from build123d import *

# Parameters (mm, degrees)
F0_W            = 12.2174
F0_H            = 38.1762
F1_DEPTH        = 117.475
F2_W            = 2.286
F2_H            = 1.778
F3_DEPTH        = 117.476
F5_DEPTH        = 117.476
F7_D            = 2.7051
F10_D           = 2.7051
F10_DEPTH       = 5.55625
F10_TIP         = 0.8126940303
F10_ON_F9_D     = 2.7051
F10_ON_F9_DEPTH = 5.55625
F10_ON_F9_TIP   = 0.8126940303


with BuildPart() as f1:
    # F0 (on Front) → F1 (new body)
    with BuildSketch(Plane.XZ):
        with Locations((6.1087, 19.0881)):
            Rectangle(F0_W, F0_H)
    extrude(amount=F1_DEPTH)

    # F2 (on face) → F3 (cut, through all)
    with BuildSketch(Plane.XZ.offset(117.475)):
        with Locations((1.143, 29.5021)):
            Rectangle(F2_W, F2_H)
        with Locations((1.143, 25.6921)):
            Rectangle(F2_W, F2_H)
        with Locations((1.143, 8.6741)):
            Rectangle(F2_W, F2_H)
        with Locations((1.143, 12.4841)):
            Rectangle(F2_W, F2_H)
    extrude(amount=-F3_DEPTH, mode=Mode.SUBTRACT)

    # F4 (on face) → F5 (cut, through all)
    with BuildSketch(Plane.XZ.offset(117.475)):
        Polygon((10.5664, 20.3581), (12.2174, 20.3581), (12.2174, 38.1762), (7.1374, 38.1762), (7.1374, 36.6522), (10.5664, 36.6522), (10.5664, 24.8031), (5.8674, 24.8031), (5.8674, 22.2631), (10.5664, 22.2631), align=None)
        Polygon((10.5664, 13.3731), (10.5664, 1.524), (7.1374, 1.524), (7.1374, 0), (12.2174, 0), (12.2174, 17.8181), (10.5664, 17.8181), (10.5664, 15.9131), (5.8674, 15.9131), (5.8674, 13.3731), align=None)
    extrude(amount=-F5_DEPTH, mode=Mode.SUBTRACT)

    # F7 (through all)
    with Locations(Plane.XZ.offset(117.475)):
        with Locations((3.2004, 34.9631), (3.2004, 3.2131)):
            Hole(F7_D / 2)

    # F10
    with Locations(Plane.YZ.offset(10.5664)):
        with Locations((-101.6, 28.3083), (-15.875, 28.3083)):
            Hole(F10_D / 2, depth=F10_DEPTH)
            with Locations((0, 0, -(F10_DEPTH + F10_TIP / 2))):  # 118° drill point
                Cone(0, F10_D / 2, F10_TIP, mode=Mode.SUBTRACT)

    # F10 on F9
    with Locations(Plane.YZ.offset(10.5664)):
        with Locations((-15.875, 9.8679), (-101.6, 9.8679)):
            Hole(F10_ON_F9_D / 2, depth=F10_ON_F9_DEPTH)
            with Locations((0, 0, -(F10_ON_F9_DEPTH + F10_ON_F9_TIP / 2))):  # 118° drill point
                Cone(0, F10_ON_F9_D / 2, F10_ON_F9_TIP, mode=Mode.SUBTRACT)


solid = f1.part
Part model, mm, in its own coordinate system. A direction names the side the tool comes from. Coordinates: 2 decimals unless noted, no trailing zeros. Order: outer loops, then holes, each group sorted by start corner. A loop starts at its lowest first (then second) coordinate and runs counter-clockwise, first axis right, second up. Notation, with made-up numbers: M 61,81 L 108,81 A24 ccw 108,100 Z; hole C -17,53.5 d10. An arc over 180 degrees is marked long. One line per question, with ' | ' between items.
Q1. Two-plate mould, pull along Z, no slides. Class faces 6 (the face through (10.566, -60, 31)), 7 (the face through (3.49, -57.92, 1.89)), 8 (the face through (4, -58, 0)): +Z half, -Z half, draft (parallel to the pull), parting line (faces both ways), or undercut.
A:
face 6: draft | face 7: undercut | face 8: -Z half
Q2. 3-axis set-ups, long thin cutter, end or side, ignore diameter. For faces 1 (the face through (7.749, -14.524, 9.927)), 2 (the face through (9, -60, 1.524)), 3 (the face through (8, -60, 24.803)), 4 (the face through (9, -60, 36.652)), 5 (the face through (1, -60, 28.613)): which of +Z, -Z, +X, -X, +Y, -Y reach the whole face in a straight line?
A:
face 1: +X | face 2: -Z, +X, +Y, -Y | face 3: +X, +Y, -Y | face 4: +Z, +X, +Y, -Y | face 5: -X, +Y, -Y
Q3. Slice it at A-A (x = 8.25). Give the cut face in (y, z) (3 decimals).
A:
outline: M -117.475,1.524 L 0,1.524 L 0,13.373 L -117.475,13.373 Z; M -117.475,15.913 L 0,15.913 L 0,22.263 L -117.475,22.263 Z; M -117.475,24.803 L 0,24.803 L 0,36.652 L -117.475,36.652 Z; hole C -101.6,9.868 d2.705; hole C -101.6,28.308 d2.705; hole C -15.875,9.868 d2.705; hole C -15.875,28.308 d2.705
Q4. Drill centre lines: line 1 (Z direction, x = 7, y = -9); line 2 (Z direction, x = 1.5, y = -24); line 3 (Z direction, x = 8.5, y = -59.5). Where is each one in solid material? Low to high.
A:
line 1: z = 0 to 13.37, 15.91 to 22.26, 24.8 to 38.18 | line 2: z = 0 to 7.79, 9.56 to 11.6, 13.37 to 24.8, 26.58 to 28.61, 30.39 to 38.18 | line 3: z = 1.52 to 13.37, 15.91 to 22.26, 24.8 to 36.65
Q5. Slice it at B-B (y = -99). Count the separate pieces of the cut face and the enclosed holes in it, and give its area (3 significant figures).
A:
separate pieces: 1 | enclosed holes: 2 | area: 346 mm^2
Q6. Pin check, flat tips, straight feed: P1, Ø4, axis at x = 6, z = 18.5, coming from the +Y side; P2, Ø0.8, axis at y = -65.5, z = 38, coming from the +X side; P3, Ø1.6, axis at x = 3.2, z = 34.96, coming from the -Y side; P4, Ø0.8, axis at y = -77.5, z = 14, coming from the +X side. Stop position of each tip, or through.
A:
P1: stops at y = 0 | P2: stops at x = 7.14 | P3: passes through | P4: stops at x = 5.87
